Check sheet for the drawn part. Datum: minimum x, y, z corner. Units: mm. A direction names the side the tool comes from. Round coordinates to 2 decimals unless told otherwise and drop trailing zeros. Loops run counter-clockwise (first coordinate to the right, second up) from the corner with the lowest first, then second, coordinate; pieces in that order, holes last. Notation, with made-up numbers: (28, 63.25) - (78, 63.25) arc R20 ccw to (78, 82.25) - close; hole circle Ø7 at (75, -14). An arc over 180 degrees is marked (long way). Use CSV: the item, a comma, the result in double quotes.
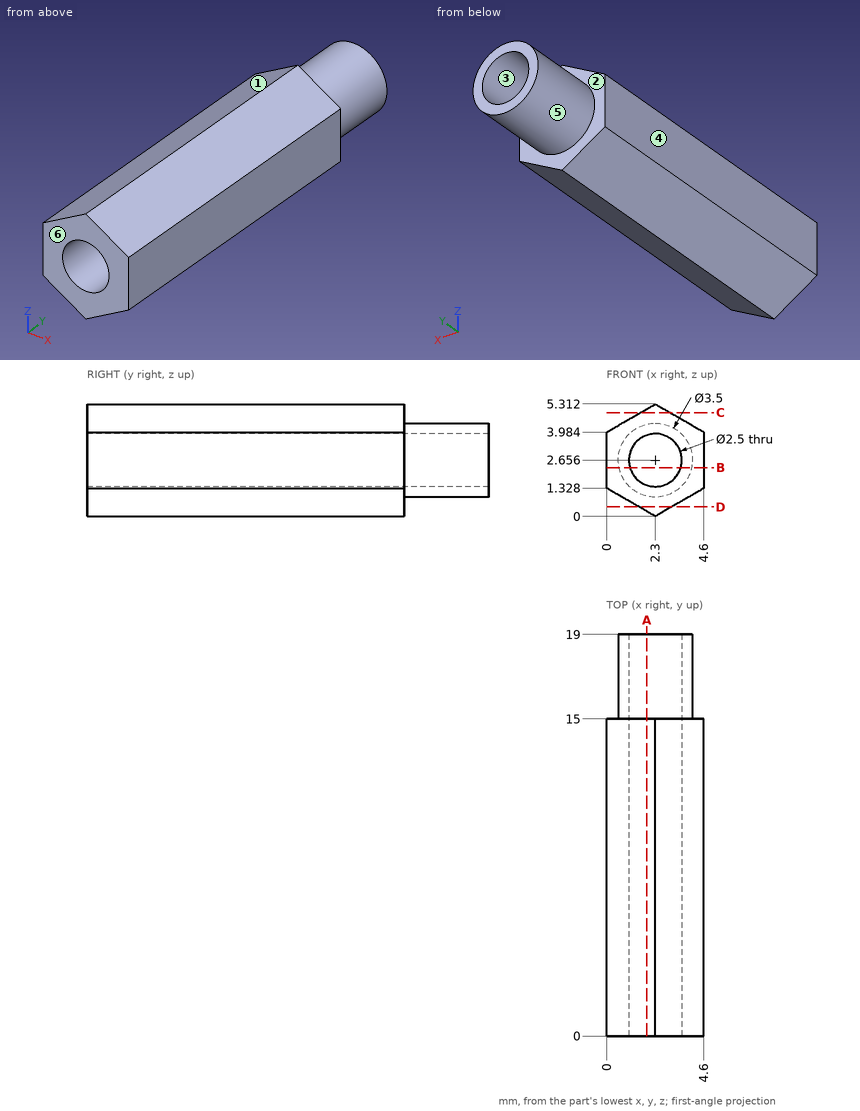
1) Access from +Z, -Z, +X, -X, +Y, -Y to the whole of each face (thin tool, end or side, straight path). Record for the marked faces 1 and 2.
Returned:
face 1,"+Z, -X, +Y, -Y"
face 2,"+Y"
2) Cross-section at C-C, the plane z = 4.9. Record the cut outline in (x, y), then the cut area to 3 significant figures.
Returned:
outline,"(1.59, 0) - (3.01, 0) - (3.01, 15) - (1.59, 15) - close"
area,"21.4 mm²"
3) Mould release check, pull along X, two halves, no side actions. Record for the marked faces 3, 4, 5 and 6: +X half, -X half, draft (parallel to the pull), parting line (faces both ways), or undercut.
Returned:
face 3,"undercut"
face 4,"-X half"
face 5,"parting line"
face 6,"draft"
4) Cross-section at D-D, the plane z = 0.45. Record the cut outline in (x, y).
Returned:
outline,"(1.52, 0) - (3.08, 0) - (3.08, 15) - (1.52, 15) - close"
5) Gauge pin test, flat ends, axial feed: pin 1 Ø1 at (x, y) = (1.5, 8.5) entering from +Z; pin 2 Ø1 at (y, z) = (9.5, 0.5) entering from -X; pin 3 Ø2 at (x, z) = (2.3, 2.66) entering from -Y. Record the tip position at first contact, or that the pin passes through.
Returned:
pin 1,"stops at z = 5.14"
pin 2,"stops at x = 0.57"
pin 3,"passes through"
6) Thickness scan on probe 1 along Y at (x, z) = (2.7, 0.6); probe 2 along Z at (x, y) = (2.6, 14.5); probe 3 along X at (y, z) = (18.25, 2.05) (1 decimal). Record the ranges inside material, lowest first. Write a range as [from, to].
Returned:
probe 1,"y = [0, 15]"
probe 2,"z = [0.17, 1.44], [3.87, 5.14]"
probe 3,"x = [0.7, 1.2], [3.4, 3.9]"
7) Cross-section at A-A, the plane x = 1.9. Record the cut outline in (y, z).
Returned:
outline,"(0, 0.23) - (15, 0.23) - (15, 0.95) - (19, 0.95) - (19, 1.47) - (0, 1.47) - close; (0, 3.84) - (19, 3.84) - (19, 4.36) - (15, 4.36) - (15, 5.08) - (0, 5.08) - close"
8) Cross-section at B-B, the plane z = 2.3. Record the cut outline in (x, y).
Returned:
outline,"(0, 0) - (1.1, 0) - (1.1, 19) - (0.59, 19) - (0.59, 15) - (0, 15) - close; (3.5, 0) - (4.6, 0) - (4.6, 15) - (4.01, 15) - (4.01, 19) - (3.5, 19) - close"
